from build123d import *

# Parameters (mm, degrees)
SKETCH047_R  = 3.1
PAD039_DEPTH = 2.8
SKETCH048_R  = 3.1
PAD040_DEPTH = 2.8
FILLET_R     = 1


with BuildPart() as part:
    # Sketch047 (on DatumPlane) → Pad039 (new body)
    with BuildSketch(Plane.YZ.offset(30.1)):
        with BuildLine():
            ThreePointArc((-25.197793, -37.709891), (-32.374027, -51.397583), (-19.31538, -43.131811))
            Line((13.245686, -7.805279), (-19.31538, -43.131811))
            ThreePointArc((13.245686, -7.805279), (20.42192, 5.882413), (7.363273, -2.383359))
            Line((-25.197793, -37.709891), (7.363273, -2.383359))
        make_face()
        with Locations((-26.952107, -45.51517)):
            Circle(SKETCH047_R, mode=Mode.SUBTRACT)
        with Locations((15, 0)):
            Circle(SKETCH047_R, mode=Mode.SUBTRACT)
    extrude(amount=PAD039_DEPTH)

    # Sketch048 (on Face8 of Pad039) → Pad040 (join)
    with BuildSketch(Plane.YZ.offset(32.9)):
        Polygon((-38.25644, -45.975663), (-26.491614, -56.819503), (-15.647774, -45.054677), (-27.4126, -34.210837), align=None)
        with Locations((-26.952107, -45.51517)):
            Circle(SKETCH048_R, mode=Mode.SUBTRACT)
    extrude(amount=-PAD040_DEPTH)

    # Fillet
    fillet_edges = [part.edges().sort_by_distance(p)[0] for p in [
        (31.5, -27.4126, -34.210837),
        (31.5, -38.25644, -45.975663),
        (31.5, -26.491614, -56.819503),
        (31.5, -15.647774, -45.054677),
        (31.5, -18.588981, -42.343717),
        (31.5, -24.471393, -36.921797),
    ]]
    fillet(fillet_edges, radius=FILLET_R)


solid = part.part
Source: CAD feature listing. Evaluate the final solid. Frame: model axes, mm. A direction names the side the tool comes from. Give positions to 0.01 mm unless a question says otherwise; leave off trailing zeros. Write each loop counter-clockwise with the first axis right and the second up, starting at its lowest first coordinate (ties: lowest second). Pieces come first, ordered by that corner, then holes. Notation, with made-up numbers: M 62.5,-35.75 L 92.5,-35.75 A20 ccw 92.5,-29.75 Z; hole C -34,4 d11. An arc over 180 degrees is marked long. Return JSON: item names as keys, results as strings. Group by question number.
1) Cut plane A-A, the plane y = 15. Output: boundary loops of the cut face in (x, z).
2) Cut plane C-C, the plane x = 31.35. Output: boundary loops of the cut face in (y, z).
3) Cut plane B-B, the plane z = 0. Output: boundary loops of the cut face in (x, y), plus the area to 3 significant figures.
4) Pull-direction query (Z, two-part tool) for faces 1 (the face through (31.48, -24.5, -36.51)), 2 (the face through (31.52, -21.136, -51.009)), 3 (the face through (31.48, -29.412, -47.401)); classes: pulls with the +Z half, pulls with the -Z half, needs draft (parallel to the pull), parting line crosses it, or undercut.
5) Set-up query: faces 4 (the face through (31.52, -17.108, -43.709)), 5 (the face through (31.52, -25.93, -35.58)), 6 (the face through (32.9, -8, -26)). Return all of +Z, -Z, +X, -X, +Y, -Y with unobstructed straight access to the full face (end or side cutting, diameter ignored); none if empty.
6) Material intervals for line 1 along Z through (x, y) = (31.65, 15); line 2 along Y through (x, z) = (32.4, -36); line 3 along Z through (x, y) = (31.95, -3), sorted ascending. Write a range as [from, to].
7) Cut plane D-D, the plane y = -22.5. Output: boundary loops of the cut face in (x, z), plus the area to 3 significant figures.
8) Pin query (flat end, axial travel): P1, Ø5, axis at y = -26.95, z = -45.52, coming from the +X side; P2, Ø1, axis at x = 31.5, z = 1, coming from the -Y side. Return the tip coordinate at first contact, or that it passes through.
Recorded:
{
 "1": {"outline": "M 30.1,-8 L 32.9,-8 L 32.9,-3.1 L 30.1,-3.1 Z; M 30.1,3.1 L 32.9,3.1 L 32.9,8 L 30.1,8 Z"},
 "2": {"outline": "M -37.58,-45.24 A1 ccw -37.52,-46.65 L -27.23,-56.14 A1 ccw -25.81,-56.08 L -16.33,-45.79 A1 ccw -16.38,-44.38 L -17.85,-43.02 A1 cw -17.91,-41.61 L 13.25,-7.81 A8 ccw long 7.36,-2.38 L -23.79,-36.19 A1 cw -25.21,-36.24 L -26.68,-34.89 A1 ccw -28.09,-34.95 Z; hole C -26.95,-45.52 d6.2; hole C 15,0 d6.2"},
 "3": {"outline": "M 30.1,7 L 32.9,7 L 32.9,11.9 L 30.1,11.9 Z; M 30.1,18.1 L 32.9,18.1 L 32.9,23 L 30.1,23 Z", "area": "27.4 mm²"},
 "4": {"face 1": "pulls with the +Z half", "face 2": "pulls with the -Z half", "face 3": "undercut"},
 "5": {"face 4": "+X, -X, +Y", "face 5": "+Z, +X, -X", "face 6": "+Z, -Z, +X, +Y, -Y"},
 "6": {"line 1": "z = [-8, -3.1], [3.1, 8]", "line 2": "y = [-29.06, -25.47], [-23.62, -12.74]", "line 3": "z = [-25.43, -13.63]"},
 "7": {"outline": "M 30.1,-52.49 L 32.9,-52.49 L 32.9,-34.78 L 30.1,-34.78 Z", "area": "49.6 mm²"},
 "8": {"P1": "passes through", "P2": "stops at y = 7.02"}
}
